Geometry check sheet. Reference: the model listing, model coordinates, mm. A direction names the side the tool comes from. Coordinates: 2 decimals unless noted, no trailing zeros. Write each loop counter-clockwise with the first axis right and the second up, starting at its lowest first coordinate (ties: lowest second). Pieces come first, ordered by that corner, then holes.
from build123d import *

# Parameters (mm, degrees)
SKETCH2_W           = 120
SKETCH2_H           = 250
BOSS_EXTRUDE1_DEPTH = 100
CUT_EXTRUDE1_DEPTH  = 295.78805946
SKETCH4_OUTSIDE_W   = 310.958
SKETCH4_OUTSIDE_H   = 160.958
SKETCH4_OUTSIDE_R   = 25
CUT_EXTRUDE2_DEPTH  = 295.78805946
CUT_EXTRUDE6_DEPTH  = 60
SKETCH5_4_R         = 25
BOSS_EXTRUDE3_DEPTH = 120
SKETCH6_W           = 60
SKETCH6_H           = 17.4
CUT_EXTRUDE7_DEPTH  = 0.1
SKETCH7_W           = 60
SKETCH7_H           = 17.4
CUT_EXTRUDE8_DEPTH  = 0.1
SKETCH8_W           = 60
SKETCH8_H           = 17.4
CUT_EXTRUDE9_DEPTH  = 0.1
FILLET5_R           = 12
FILLET6_R           = 12


with BuildPart() as part:
    # Sketch2 → Boss-Extrude1 (new body)
    with BuildSketch(Plane(origin=(0, 0, 0), x_dir=(0, 1, 0), z_dir=(0, 0, 1))):
        with Locations((-60, 125)):
            Rectangle(SKETCH2_W, SKETCH2_H)
    extrude(amount=BOSS_EXTRUDE1_DEPTH)

    # Sketch3 → Cut-Extrude1 (cut, through all)
    with BuildSketch(Plane.XY.offset(100)):
        with BuildLine():
            Line((-179.498344353, -90), (-250, -90))
            Line((-250, -90), (-250, -120))
            Line((-250, -120), (-103.999999784, -120))
            ThreePointArc((-103.999999784, -120), (-126.156468276, -115.759222677), (-145.180915101, -103.636363636))
            ThreePointArc((-145.180915101, -103.636363636), (-161.034620706, -93.533981136), (-179.498344353, -90))
        make_face()
        with BuildLine():
            Line((-250, 0), (-250, -30))
            Line((-250, -30), (-179.498344353, -30))
            ThreePointArc((-179.498344353, -30), (-161.034620706, -26.466018864), (-145.180915101, -16.363636364))
            ThreePointArc((-145.180915101, -16.363636364), (-126.156468376, -4.240777363), (-104, 0))
            Line((-104, 0), (-250, 0))
        make_face()
        with BuildLine():
            Line((-44, -60), (-130, -60))
            ThreePointArc((-130, -60), (-121.213203436, -81.213203436), (-100, -90))
            Line((-100, -90), (-52.038475773, -90))
            ThreePointArc((-52.038475773, -90), (-46.044450423, -75.529142706), (-44, -60))
        make_face()
        with BuildLine():
            ThreePointArc((-100, -30), (-121.213203436, -38.786796564), (-130, -60))
            Line((-130, -60), (-44, -60))
            ThreePointArc((-44, -60), (-46.044450423, -44.470857294), (-52.038475773, -30))
            Line((-52.038475773, -30), (-100, -30))
        make_face()
        with BuildLine():
            Line((0, -60), (-44, -60))
            ThreePointArc((-44, -60), (-46.044450423, -75.529142706), (-52.038475773, -90))
            Line((-52.038475773, -90), (0, -90))
            Line((0, -90), (0, -60))
        make_face()
        with BuildLine():
            ThreePointArc((-52.038475773, -30), (-46.044450423, -44.470857294), (-44, -60))
            Line((-44, -60), (0, -60))
            Line((0, -60), (0, -30))
            Line((0, -30), (-52.038475773, -30))
        make_face()
    extrude(amount=-CUT_EXTRUDE1_DEPTH, mode=Mode.SUBTRACT)

    # Sketch4 outside → Cut-Extrude2 (cut, through all)
    # profile 1 of 2: a face of its own
    with BuildSketch(Plane(origin=(0, 0, 0), x_dir=(-1, 0, 0), z_dir=(0, 1, 0))):
        with Locations((125, 50)):
            Rectangle(SKETCH4_OUTSIDE_W, SKETCH4_OUTSIDE_H)
        with BuildLine():
            Line((250, 80), (100.990195136, 80))
            ThreePointArc((100.990195136, 80), (91.861485844, 81.726266594), (83.993463424, 86.666666667))
            ThreePointArc((83.993463424, 86.666666667), (0, 50), (83.993463424, 13.333333333))
            ThreePointArc((83.993463424, 13.333333333), (91.861485844, 18.273733406), (100.990195136, 20))
            Line((100.990195136, 20), (250, 20))
            Line((250, 20), (250, 80))
        make_face(mode=Mode.SUBTRACT)
    # profile 2 of 2: a face of its own
    with BuildSketch(Plane(origin=(0, 0, 0), x_dir=(-1, 0, 0), z_dir=(0, 1, 0))):
        with Locations(Location((50, 50, 0), (0, 0, 90))):
            Circle(SKETCH4_OUTSIDE_R)
    extrude(amount=-CUT_EXTRUDE2_DEPTH, mode=Mode.SUBTRACT)

    # Sketch5 → Cut-Extrude6 (cut)
    with BuildSketch(Plane(origin=(-250, 0, 0), x_dir=(0, -1, 0), z_dir=(-1, 0, 0))):
        Polygon((72.6, 80), (90, 62.6), (90, 80), align=None)
        Polygon((72.608172947, 20.008172947), (90.008172947, 20.008172947), (90.008172947, 37.408172947), align=None)
        Polygon((30.016345893, 37.4), (30.016345893, 20), (47.416345893, 20), align=None)
        Polygon((47.408172947, 79.991827053), (30.008172947, 79.991827053), (30.008172947, 62.591827053), align=None)
    extrude(amount=-CUT_EXTRUDE6_DEPTH, mode=Mode.SUBTRACT)

    # Sketch5_4 → Boss-Extrude3 (add)
    with BuildSketch(Plane(origin=(-250, 0, 0), x_dir=(0, -1, 0), z_dir=(-1, 0, 0))):
        with Locations(Location((60.008172947, 50, 0), (0, 0, 180))):
            Circle(SKETCH5_4_R)
    extrude(amount=BOSS_EXTRUDE3_DEPTH)

    # Sketch6 → Cut-Extrude7 (cut)
    with BuildSketch(Plane(origin=(0, -30, 0), x_dir=(1, 0, 0), z_dir=(0, 1, 0))):
        with Locations((-220, -71.3)):
            Rectangle(SKETCH6_W, SKETCH6_H)
        with Locations((-220, -28.7)):
            Rectangle(SKETCH6_W, SKETCH6_H)
    extrude(amount=-CUT_EXTRUDE7_DEPTH, mode=Mode.SUBTRACT)

    # Sketch7 → Cut-Extrude8 (cut)
    with BuildSketch(Plane(origin=(0, 0, 20), x_dir=(-1, 0, 0), z_dir=(0, 0, -1))):
        with Locations((220, -81.3)):
            Rectangle(SKETCH7_W, SKETCH7_H)
    extrude(amount=-CUT_EXTRUDE8_DEPTH, mode=Mode.SUBTRACT)

    # Sketch8 → Cut-Extrude9 (cut)
    with BuildSketch(Plane.XY.offset(80)):
        with Locations((-220, -38.8)):
            Rectangle(SKETCH8_W, SKETCH8_H)
    extrude(amount=-CUT_EXTRUDE9_DEPTH, mode=Mode.SUBTRACT)

    # Fillet5
    fillet5_edges = [part.edges().sort_by_distance(p)[0] for p in [
        (-190, -38.708172947, 71.291827053),
    ]]
    fillet(fillet5_edges, radius=FILLET5_R)

    # Fillet6
    fillet6_edges = [part.edges().sort_by_distance(p)[0] for p in [
        (-190, -81.3, 71.3),
        (-190, -38.758172947, 28.658172947),
        (-190, -81.35, 28.75),
    ]]
    fillet(fillet6_edges, radius=FILLET6_R)


solid = part.part
1. Sectioned sample at C-C, the plane y = -7.5. Record the boundary of the cut face in (x, z), and give its area (3 significant figures).
Computed values:
outline: (-133.05, 20) - (-100.99, 20) arc R25 cw to (-83.99, 13.33) arc R50 ccw (long way) to (-83.99, 86.67) arc R25 cw to (-100.99, 80) - (-133.05, 80) - close; hole circle Ø50 at (-50, 50)
area: 8,090 mm2
2. Sectioned sample at D-D, the plane y = -69. Record the boundary of the cut face in (x, z).
Computed values:
outline: (-370, 26.67) - (-250, 26.67) - (-250, 20) - (-128.62, 20) - (-128.62, 80) - (-250, 80) - (-250, 73.33) - (-370, 73.33) - close
3. Thickness scan on line 1 along Y through (x, z) = (-24, 38.5); line 2 along Z through (x, y) = (-243.5, -56); line 3 along X through (y, z) = (-102, 50). Record the ranges inside material, lowest first.
Computed values:
line 1: y = -120 to -90, -30 to 0
line 2: z = 20 to 80
line 3: x = -147 to -75, -25 to 0
4. Access from +Z, -Z, +X, -X, +Y, -Y to the whole of each face (thin tool, end or side, straight path). Record for faces 5 (the flat face through (-226.336, -38.879, 28.537)), 6 (the flat face through (-160, -59, 80)), 7 (the flat face through (-226.336, -38.588, 71.171)), 8 (the cylindrical face through (-126.45, -4.36, 50.42)), 9 (the cylindrical face through (-65, -105, 30)).
Computed values:
face 5: -Z, -X, +Y
face 6: +Z, -X, +Y, -Y
face 7: +Z, -X, +Y
face 8: +Z, -Z, -X, +Y
face 9: +Y, -Y
5. Draft check along Y on faces 1 (the flat face through (-193, -30.1, 66)), 2 (the cylindrical face through (-160.79, -93.63, 50.42)), 3 (the cylindrical face through (-91.74, -14.798, 18.226)), 4 (the flat face through (-27.1, -30, 39.6)). Enter one of: released by +Y, released by -Y, zero draft, split by the parting line, or undercut.
Computed values:
face 1: released by +Y
face 2: released by -Y
face 3: zero draft
face 4: undercut
6. Gauge pin test, flat ends, axial feed: pin 1 Ø8 at (x, z) = (-329, 47) entering from +Y; pin 2 Ø0.5 at (y, z) = (-30, 25) entering from -X; pin 3 Ø6 at (x, y) = (-131.5, -70) entering from -Z. Record the tip position at first contact, or that the pin passes through.
Computed values:
pin 1: stops at y = -35.01
pin 2: stops at x = -190.51
pin 3: stops at z = 20
7. Sectioned sample at B-B, the plane x = -50. Record the boundary of the cut face in (y, z), and give its area (3 significant figures).
Computed values:
outline: (-120, 0) - (-90, 0) - (-90, 25) - (-120, 25) - close; (-120, 75) - (-90, 75) - (-90, 100) - (-120, 100) - close; (-30, 0) - (0, 0) - (0, 25) - (-30, 25) - close; (-30, 75) - (0, 75) - (0, 100) - (-30, 100) - close
area: 3,000 mm2
8. Sectioned sample at A-A, the plane z = 50. Record the boundary of the cut face in (x, y).
Computed values:
outline: (-370, -85.01) - (-250, -85.01) - (-250, -90) - (-179.5, -90) arc R50 cw to (-145.18, -103.64) arc R60 ccw to (-104, -120) - (-75, -120) - (-75, -90) - (-100, -90) arc R30 cw to (-100, -30) - (-75, -30) - (-75, 0) - (-104, 0) arc R60 ccw to (-145.18, -16.36) arc R50 cw to (-179.5, -30) - (-250, -30) - (-250, -35.01) - (-370, -35.01) - close; (-25, -120) - (0, -120) - (0, -90) - (-25, -90) - close; (-25, -30) - (0, -30) - (0, 0) - (-25, 0) - close
